For this review, take the finished solid that the model builds, in its own axes (mm). Face numbers are marked on the shaded views. A direction names the side the tool comes from. Give positions to 0.01 mm unless a question says otherwise; leave off trailing zeros. Write each loop counter-clockwise with the first axis right and the second up, starting at its lowest first coordinate (ties: lowest second). Pieces come first, ordered by that corner, then holes. Notation, with made-up numbers: M 65.5,34.5 L 75.5,34.5 A32 cw 75.5,64.5 Z; hole C 26.5,-20.5 d10. An arc over 180 degrees is marked long. Use one line per item in the form item = value. Start each with the question number.
Q1. Consider section A-A on z = -5. Write out the cut boundary in (x, y), and give its area (3 significant figures).
Q2. Consider section D-D on x = 35. Write out the cut boundary in (y, z), and give its area (3 significant figures).
Q3. Clearance check with flat-ended pins moving along their axes: pin 1 Ø2.5 at (x, z) = (49.581, -15) entering from -Y; pin 2 Ø7 at (x, z) = (-11, -10) entering from -Y; pin 3 Ø2 at (y, z) = (17.5, -3.5) entering from +X; pin 4 Ø12 at (x, z) = (12.5, -7) entering from +Y. State where each tip first meets the part, or that it passes through.
Q4. For probe 1 along X at (y, z) = (11.5, -18.25); probe 2 along X at (y, z) = (20.1, -5); probe 3 along X at (y, z) = (19.75, -15), list the stretches that pass through material, from the lowest coordinate up. Write a range as [from, to].
Q5. Consider section B-B on y = 10.25. Write out the cut boundary in (x, z), and give its area (3 significant figures).
Q6. Mouldability with a two-part tool opening along X and no side actions: class the marked faces 1, 2 and 3 as released by +X, released by -X, zero draft, split by the parting line, or undercut.
Q7. Tool access review of the marked faces 4, 5 and 6: name each direction out of +Z, -Z, +X, -X, +Y, -Y from which nothing blocks a thin tool from reaching the whole face with its end or side.
Q8. Consider section C-C on z = -10.5. Write out the cut boundary in (x, y), and give its area (3 significant figures).
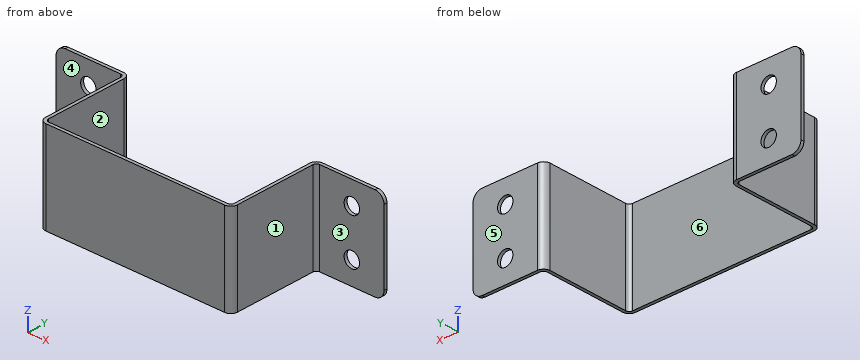
```python
from build123d import *

# Parameters (mm, degrees)
SKETCH1_W                    = 41
SKETCH1_H                    = 20
BASE_FLANGE1_DEPTH           = 0.7
EDGE_FLANGE1_STRIP_W         = 4.324
EDGE_FLANGE1_STRIP_H         = 0.7
EDGE_FLANGE1_STRIP_CUT_DEPTH = 20
EDGE_FLANGE1_DEPTH           = 20
EDGE_FLANGE2_STRIP_W         = 4.324
EDGE_FLANGE2_STRIP_H         = 0.7
EDGE_FLANGE2_STRIP_CUT_DEPTH = 20
EDGE_FLANGE2_DEPTH           = 20
EDGE_FLANGE3_STRIP_W         = 4.324
EDGE_FLANGE3_STRIP_H         = 0.7
EDGE_FLANGE3_STRIP_CUT_DEPTH = 20
EDGE_FLANGE3_DEPTH           = 20
M3_CLEARANCE_HOLE1_D         = 3.4
M3_CLEARANCE_HOLE1_DEPTH     = 3
M3_CLEARANCE_HOLE1_TIP       = 1.021463052
FILLET1_R                    = 2


# Sheet-metal steps are written as plain solids
with BuildPart() as part:
    # Sketch1 → Base-Flange1 (new body)
    with BuildSketch(Plane(origin=(0, 0, 0), x_dir=(1, 0, 0), z_dir=(0, 1, 0))):
        with Locations((20.5, 10)):
            Rectangle(SKETCH1_W, SKETCH1_H)
    extrude(amount=-BASE_FLANGE1_DEPTH)

    # Edge-Flange1 strip (across the edge) → Edge-Flange1 strip cut (cut)
    with BuildSketch(Plane(origin=(41, 0, 0), x_dir=(-1, 0, 0), z_dir=(0, 0, -1))):
        with Locations((-1.4, -0.35)):
            Rectangle(EDGE_FLANGE1_STRIP_W, EDGE_FLANGE1_STRIP_H)
    extrude(amount=EDGE_FLANGE1_STRIP_CUT_DEPTH, mode=Mode.SUBTRACT)

    # Edge-Flange1 section (across the edge) → Edge-Flange1 (add)
    with BuildSketch(Plane(origin=(41, 0, 0), x_dir=(-1, 0, 0), z_dir=(0, 0, -1))):
        with BuildLine():
            Line((-0.7, 0.762), (-0.7, 20.25))
            Line((-0.7, 20.25), (0, 20.25))
            Line((0, 20.25), (0, 0.762))
            ThreePointArc((0, 0.762), (0.223184633, 0.223184633), (0.762, 0))
            Line((0.762, 0), (0.762, -0.7))
            ThreePointArc((0.762, -0.7), (-0.271790114, -0.271790114), (-0.7, 0.762))
        make_face()
    extrude(amount=EDGE_FLANGE1_DEPTH)

    # Edge-Flange2 strip (across the edge) → Edge-Flange2 strip cut (cut)
    with BuildSketch(Plane(origin=(41.7, 20.25, -20), x_dir=(0, -1, 0), z_dir=(0, 0, 1))):
        with Locations((-0.7, -0.35)):
            Rectangle(EDGE_FLANGE2_STRIP_W, EDGE_FLANGE2_STRIP_H)
    edge_flange2_strip_cut = extrude(amount=EDGE_FLANGE2_STRIP_CUT_DEPTH, mode=Mode.SUBTRACT)

    # Edge-Flange2 section (across the edge) → Edge-Flange2 (add)
    with BuildSketch(Plane(origin=(41.7, 20.25, -20), x_dir=(0, -1, 0), z_dir=(0, 0, 1))):
        with BuildLine():
            Line((0, 0.762), (0, 15))
            Line((0, 15), (0.7, 15))
            Line((0.7, 15), (0.7, 0.762))
            ThreePointArc((0.7, 0.762), (0.923184633, 0.223184633), (1.462, 0))
            Line((1.462, 0), (1.462, -0.7))
            ThreePointArc((1.462, -0.7), (0.428209886, -0.271790114), (0, 0.762))
        make_face()
    edge_flange2 = extrude(amount=EDGE_FLANGE2_DEPTH)

    # Edge-Flange3 strip (across the edge) → Edge-Flange3 strip cut (cut)
    with BuildSketch(Plane.XY.offset(-20)):
        with Locations((-1.4, -0.35)):
            Rectangle(EDGE_FLANGE3_STRIP_W, EDGE_FLANGE3_STRIP_H)
    extrude(amount=EDGE_FLANGE3_STRIP_CUT_DEPTH, mode=Mode.SUBTRACT)

    # Edge-Flange3 section (across the edge) → Edge-Flange3 (add)
    with BuildSketch(Plane.XY.offset(-20)):
        with BuildLine():
            Line((-0.7, 0.762), (-0.7, 20.25))
            Line((-0.7, 20.25), (0, 20.25))
            Line((0, 20.25), (0, 0.762))
            ThreePointArc((0, 0.762), (0.223184633, 0.223184633), (0.762, 0))
            Line((0.762, 0), (0.762, -0.7))
            ThreePointArc((0.762, -0.7), (-0.271790114, -0.271790114), (-0.7, 0.762))
        make_face()
    extrude(amount=EDGE_FLANGE3_DEPTH)

    # Mirror2: Edge-Flange2 strip cut, Edge-Flange2 across plane
    add(edge_flange2_strip_cut.mirror(Plane(origin=(20.5, 0, 0), x_dir=(0, 0, 1), z_dir=(1, 0, 0))), mode=Mode.SUBTRACT)
    add(edge_flange2.mirror(Plane(origin=(20.5, 0, 0), x_dir=(0, 0, 1), z_dir=(1, 0, 0))))

    # M3 Clearance Hole1
    with Locations(Plane(origin=(0, 20.25, 0), x_dir=(1, 0, 0), z_dir=(0, 1, 0))):
        with Locations((49.581, 5), (49.581, 15), (-8.581, 15), (-8.581, 5)):
            Hole(M3_CLEARANCE_HOLE1_D / 2, depth=M3_CLEARANCE_HOLE1_DEPTH)
            with Locations((0, 0, -(M3_CLEARANCE_HOLE1_DEPTH + M3_CLEARANCE_HOLE1_TIP / 2))):  # 118° drill point
                Cone(0, M3_CLEARANCE_HOLE1_D / 2, M3_CLEARANCE_HOLE1_TIP, mode=Mode.SUBTRACT)

    # Fillet1
    fillet1_edges = [part.edges().sort_by_distance(p)[0] for p in [
        (-15.7, 19.9, 0),
        (-15.7, 19.9, -20),
        (56.7, 19.9, -20),
        (56.7, 19.9, 0),
    ]]
    fillet(fillet1_edges, radius=FILLET1_R)


solid = part.part
```
Working result:
q1.outline = M -15.7,19.55 L -10.28,19.55 L -10.28,20.25 L -15.7,20.25 Z; M -6.88,19.55 L -1.46,19.55 A0.76 cw -0.7,18.79 L -0.7,0.76 A1.46 ccw 0.76,-0.7 L 40.24,-0.7 A1.46 ccw 41.7,0.76 L 41.7,18.79 A0.76 cw 42.46,19.55 L 47.88,19.55 L 47.88,20.25 L 42.46,20.25 A1.46 ccw 41,18.79 L 41,0.76 A0.76 cw 40.24,0 L 0.76,0 A0.76 cw 0,0.76 L 0,18.79 A1.46 ccw -1.46,20.25 L -6.88,20.25 Z; M 51.28,19.55 L 56.7,19.55 L 56.7,20.25 L 51.28,20.25 Z
q1.area = 72.9 mm²
q2.outline = M -0.7,-20 L 0,-20 L 0,0 L -0.7,0 Z
q2.area = 14.0 mm²
q3.pin_1 = through
q3.pin_2 = 19.55
q3.pin_3 = 41.7
q3.pin_4 = 0
q4.probe_1 = [-0.7, 0], [41, 41.7]
q4.probe_2 = [-15.7, -10.28], [-6.88, -0.82], [41.82, 47.88], [51.28, 56.7]
q4.probe_3 = [-15.7, -10.28], [-6.88, -0.36], [41.36, 47.88], [51.28, 56.7]
q5.outline = M -0.7,-20 L 0,-20 L 0,0 L -0.7,0 Z; M 41,-20 L 41.7,-20 L 41.7,0 L 41,0 Z
q5.area = 28.0 mm²
q6.face_1 = released by +X
q6.face_2 = undercut
q6.face_3 = zero draft
q7.face_4 = +Z, -Z, -X, -Y
q7.face_5 = +Z, -Z, +X, -X, +Y
q7.face_6 = +Z, -Z, +Y
q8.outline = M -15.7,19.55 L -1.46,19.55 A0.76 cw -0.7,18.79 L -0.7,0.76 A1.46 ccw 0.76,-0.7 L 40.24,-0.7 A1.46 ccw 41.7,0.76 L 41.7,18.79 A0.76 cw 42.46,19.55 L 56.7,19.55 L 56.7,20.25 L 42.46,20.25 A1.46 ccw 41,18.79 L 41,0.76 A0.76 cw 40.24,0 L 0.76,0 A0.76 cw 0,0.76 L 0,18.79 A1.46 ccw -1.46,20.25 L -15.7,20.25 Z
q8.area = 77.7 mm²
